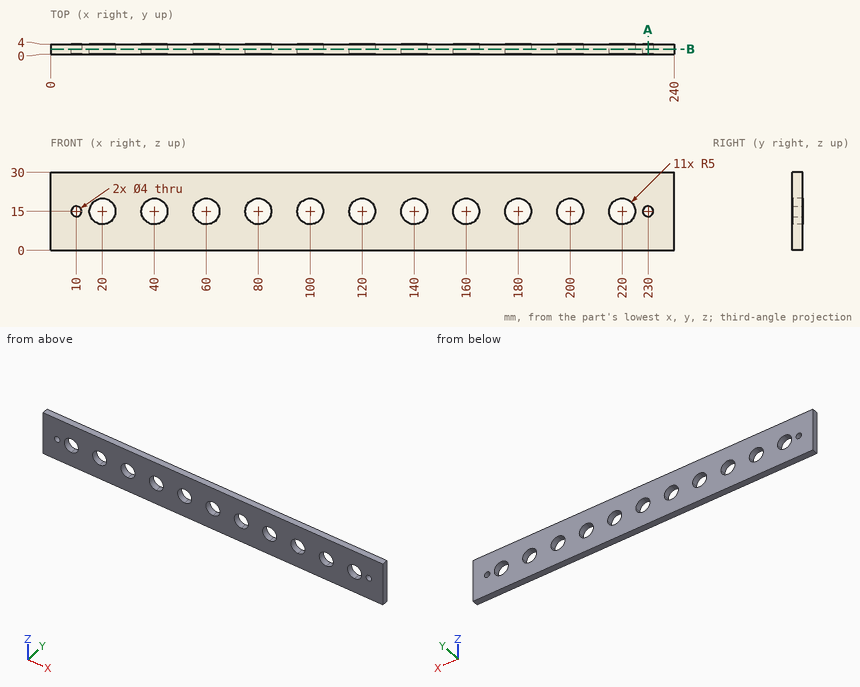
Verification items for this drawing (mm, ordinates from the low corner). Round coordinates to 2 decimals unless told otherwise and drop trailing zeros. Order: outer loops, then holes, each group sorted by start corner. A loop starts at its lowest first (then second) coordinate and runs counter-clockwise, first axis right, second up.
1) Cross-section at A-A, the plane x = 230. Record the cut outline in (y, z), plus the area to 3 significant figures.
Geometry says:
outline: (0, 0) - (4, 0) - (4, 13) - (0, 13) - close; (0, 17) - (4, 17) - (4, 30) - (0, 30) - close
area: 104 mm2
2) Material ranges on line 1 (Z direction, x = 10, y = 1.9); line 2 (Z direction, x = 20, y = 3.45), recorded low to high.
Geometry says:
line 1: z = 0 to 13, 17 to 30
line 2: z = 0 to 10, 20 to 30
3) Cross-section at B-B, the plane y = 2. Give the number of separate pieces and of enclosed holes in the cut face, plus the area to 3 significant figures.
Geometry says:
separate pieces: 1
enclosed holes: 13
area: 6,310 mm2
